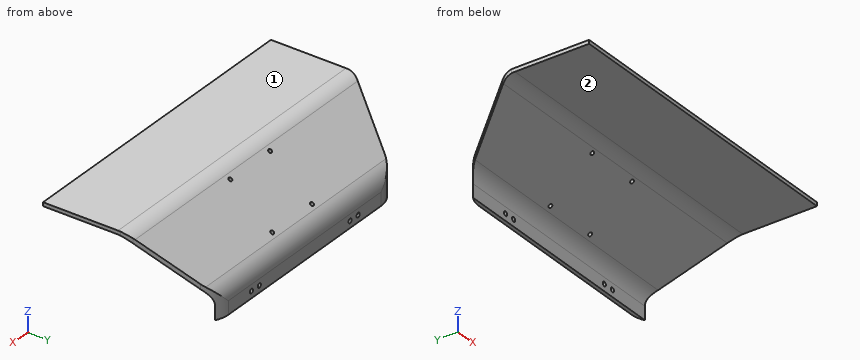
from build123d import *

# Parameters (mm, degrees)
SALIENTE_EXTRUIR1_DEPTH = 126
REDONDEO1_R             = 18
REDONDEO2_R             = 20
REDONDEO3_R             = 17
REDONDEO4_R             = 17
CORTAR_EXTRUIR1_DEPTH   = 186.234557368
REDONDEO5_R             = 17
CORTAR_EXTRUIR2_DEPTH   = 186.23455747
CROQUIS6_R              = 1.75
CORTAR_EXTRUIR3_DEPTH   = 20
CROQUIS7_W              = 252
CROQUIS7_H              = 3
CORTAR_EXTRUIR4_DEPTH   = 1
CROQUIS9_R              = 1.5
CORTAR_EXTRUIR5_DEPTH   = 183.297245602


with BuildPart() as part:
    # Croquis1 → Saliente-Extruir1 (new, symmetric)
    with BuildSketch(Plane(origin=(0, 0, 0), x_dir=(0, 0, -1), z_dir=(1, 0, 0))):
        Polygon((0, 0), (0, 66.908089297), (41.999818789, 116.961524227), (60.600895814, 116.961524227), (60.600895814, 119.961524227), (40.600895814, 119.961524227), (-3, 68), (-3, 0), align=None)
    extrude(amount=SALIENTE_EXTRUIR1_DEPTH, both=True)

    # Redondeo1
    redondeo1_edges = [part.edges().sort_by_distance(p)[0] for p in [
        (0, 68, 3),
    ]]
    fillet(redondeo1_edges, radius=REDONDEO1_R)

    # Redondeo2
    redondeo2_edges = [part.edges().sort_by_distance(p)[0] for p in [
        (0, 119.961524227, -40.600895814),
    ]]
    fillet(redondeo2_edges, radius=REDONDEO2_R)

    # Redondeo3
    redondeo3_edges = [part.edges().sort_by_distance(p)[0] for p in [
        (0, 116.961524227, -41.999818789),
    ]]
    fillet(redondeo3_edges, radius=REDONDEO3_R)

    # Redondeo4
    redondeo4_edges = [part.edges().sort_by_distance(p)[0] for p in [
        (0, 66.908089297, 0),
    ]]
    fillet(redondeo4_edges, radius=REDONDEO4_R)

    # Croquis2 → Cortar-Extruir1 (cut, through all)
    with BuildSketch(Plane.XY.offset(3)):
        Polygon((-96, 119.961524227), (-126, 68), (-126, 119.961524227), align=None)
    cortar_extruir1 = extrude(amount=-CORTAR_EXTRUIR1_DEPTH, mode=Mode.SUBTRACT)

    # Simetría1: Cortar-Extruir1 across plane
    add(cortar_extruir1.mirror(Plane(origin=(0, 0, 0), x_dir=(0, 0, 1), z_dir=(1, 0, 0))), mode=Mode.SUBTRACT)

    # Redondeo5
    # the kernel refuses this fillet: 17 mm, written as the material it takes off along each edge
    with BuildSketch(Plane(origin=(-126, 68, 13.153231119), x_dir=(0, -1, 0), z_dir=(0, 0, -1)), Plane(origin=(126, 68, 13.153231119), x_dir=(-0.49999999999999856, 0.8660254037844395, 0), z_dir=(0, 0, -1))) as redondeo5_piece_1:
        with BuildLine():
            CenterArc((REDONDEO5_R * 0.267949192431, -REDONDEO5_R), REDONDEO5_R, 90, 30)
            Line((-REDONDEO5_R * 0.232050807569, -REDONDEO5_R * 0.133974596216), (0, 0))
            Line((0, 0), (REDONDEO5_R * 0.267949192431, 0))
        make_face()
    extrude(amount=26.178446129, mode=Mode.SUBTRACT)

    # Croquis5 → Cortar-Extruir2 (cut, through all)
    with BuildSketch(Plane(origin=(0, 0, -60.600895814), x_dir=(-1, 0, 0), z_dir=(0, 0, -1))):
        with BuildLine():
            Line((84.452994616, 119.961524227), (96, 119.961524227))
            Line((96, 119.961524227), (101.773502692, 109.961524227))
            ThreePointArc((101.773502692, 109.961524227), (94.452994616, 117.282032303), (84.452994616, 119.961524227))
        make_face()
    cortar_extruir2 = extrude(amount=-CORTAR_EXTRUIR2_DEPTH, mode=Mode.SUBTRACT)

    # Simetría2: Cortar-Extruir2 across plane
    add(cortar_extruir2.mirror(Plane(origin=(0, 0, 0), x_dir=(0, 0, 1), z_dir=(1, 0, 0))), mode=Mode.SUBTRACT)

    # Croquis6 → Cortar-Extruir3 (cut)
    with BuildSketch(Plane(origin=(0, 119.961524227, 0), x_dir=(1, 0, 0), z_dir=(0, 1, 0))):
        with Locations(Location((-59, 55.100895814, 0), (0, 0, 270))):
            Circle(CROQUIS6_R)
        with Locations(Location((-50.2, 55.100895814, 0), (0, 0, 270))):
            Circle(CROQUIS6_R)
    cortar_extruir3 = extrude(amount=-CORTAR_EXTRUIR3_DEPTH, mode=Mode.SUBTRACT)

    # Simetría3: Cortar-Extruir3 across plane
    add(cortar_extruir3.mirror(Plane(origin=(0, 0, 0), x_dir=(0, 0, 1), z_dir=(1, 0, 0))), mode=Mode.SUBTRACT)

    # Croquis7 → Cortar-Extruir4 (cut)
    with BuildSketch(Plane.XZ):
        with Locations((0, 1.5)):
            Rectangle(CROQUIS7_W, CROQUIS7_H)
    extrude(amount=-CORTAR_EXTRUIR4_DEPTH, mode=Mode.SUBTRACT)

    # Croquis9 → Cortar-Extruir5 (cut, through all)
    with BuildSketch(Plane(origin=(0, 29.573173589, 35.243935869), x_dir=(1, 0, 0), z_dir=(0, 0.6427876096865381, 0.7660444431189791))):
        with Locations(Location((-22, 104.71412352, 0), (0, 0, 270))):
            Circle(CROQUIS9_R)
        with Locations(Location((22, 104.71412352, 0), (0, 0, 270))):
            Circle(CROQUIS9_R)
        with Locations(Location((22, 60.71412352, 0), (0, 0, 270))):
            Circle(CROQUIS9_R)
        with Locations(Location((-22, 60.71412352, 0), (0, 0, 270))):
            Circle(CROQUIS9_R)
    extrude(amount=-CORTAR_EXTRUIR5_DEPTH, mode=Mode.SUBTRACT)


solid = part.part
Model file for the job. Use its own axes, mm. Face numbers are marked on the shaded views. A direction names the side the tool comes from. Round coordinates to 2 decimals unless told otherwise and drop trailing zeros. Order: outer loops, then holes, each group sorted by start corner. A loop starts at its lowest first (then second) coordinate and runs counter-clockwise, first axis right, second up. Notation, with made-up numbers: M -18,86 L 25,86 A14 cw 25,108 Z; hole C 59.25,-34 d5. An arc over 180 degrees is marked long. Write each question's results on one line, items separated by ' | '. Start each with the question number.
(1) Drop flat-ended pins along their axis: pin 1 (18 mm diameter, centred on x = 10, y = 40.5, fed in from -Z); pin 2 (5.5 mm diameter, centred on x = -40.5, z = -55, fed in from -Y); pin 3 (6 mm diameter, centred on x = -28, y = 95.5, fed in from -Z). Give the stop position or say it passes through.
(2) Which spindle directions (+Z, -Z, +X, -X, +Y, -Y) get a long thin tool onto all of the face, cutting with end or side? Do the marked faces 1 and 2. Say none if no direction does.
(3) Saw through at A-A, the plane x = -28. Give the cut face in (y, z).
(4) Saw through at D-D, the plane x = -87.5. Give the cut face in (y, z), then the cut area to 3 significant figures.
(5) Saw through at B-B, the plane y = 17.5. Give the cut face in (x, z).
(6) Probe probe 1 along Z at (x, y) = (1, 24); probe 2 along Z at (x, y) = (50, 118); probe 3 along Z at (x, y) = (59, 118). List the from-to ranges inside material, lowest first. Write a range as from..to.
(7) Saw through at C-C, the plane z = -23.5. Give the cut face in (x, y).
Established:
1) pin 1: stops at z = 0 | pin 2: stops at y = 116.96 | pin 3: stops at z = -26.51
2) face 1: +Z, +X, -X, +Y, -Y | face 2: -Z, +X, -X, -Y
3) outline: M 1,0 L 60.72,0 A17 cw 71.65,-3.98 L 110.89,-36.9 A17 cw 116.96,-49.93 L 116.96,-60.6 L 119.96,-60.6 L 119.96,-49.93 A20 ccw 112.82,-34.61 L 73.02,-1.21 A18 ccw 61.45,3 L 1,3 Z
4) outline: M 1,0 L 60.72,0 A17 cw 71.65,-3.98 L 110.89,-36.9 A17 cw 116.96,-49.93 L 116.96,-60.6 L 119.73,-60.6 L 119.73,-46.88 A20 ccw 112.82,-34.61 L 73.02,-1.21 A18 ccw 61.45,3 L 1,3 Z | area: 450 mm^2
5) outline: M -126,0 L 126,0 L 126,3 L -126,3 Z
6) probe 1: z = 0..3 | probe 2: z = -60.6..-56.84, -53.36..-41.29 | probe 3: z = -60.6..-56.85, -53.35..-41.29
7) outline: M -110.46,94.91 L 110.46,94.91 L 107.77,99.58 L -107.77,99.58 Z
